Source: CAD feature listing. Evaluate the final solid. Frame: model axes, mm. A direction names the side the tool comes from. Round coordinates to 2 decimals unless told otherwise and drop trailing zeros. Write each loop counter-clockwise with the first axis right and the second up, starting at its lowest first coordinate (ties: lowest second). Pieces come first, ordered by that corner, then holes. Notation, with made-up numbers: M 42,87.5 L 46,87.5 A20 ccw 46,93.5 Z; hole C 78,-13.75 d3. An arc over 180 degrees is marked long. Use a Markdown table: item, result.
Autodesk Inventor part; units mm, degrees
ref_plane "YZ Plane" through (0, 0, 0) normal (1, 0, 0) x (0, 1, 0)
ref_plane "XZ Plane" through (0, 0, 0) normal (0, 1, 0) x (-1, 0, 0)
ref_plane "XY Plane" through (0, 0, 0) normal (0, 0, 1) x (1, 0, 0)
sketch "Sketch1" plane through (0, 0, 0) normal (0, 1, 0) x (-1, 0, 0)
  line L0 (-15.7, 12.7) -> (15.7, 12.7)
  line L1 (15.7, 12.7) -> (15.7, -12.7)
  line L2 (15.7, -12.7) -> (-15.7, -12.7)
  line L3 (-15.7, -12.7) -> (-15.7, 12.7)
  line L4 (-15.7, 12.7) -> (15.7, -12.7) construction
  line L5 (15.7, 12.7) -> (-15.7, -12.7) construction
  point P0 (0, 0)
  dimension "d0" = 25.4
  dimension "d1" = 31.4
extrude "Extrusion1" add sketch "Sketch1" along normal mid plane 6
sketch "Sketch2" plane through (0, 3, 0) normal (0, 1, 0) x (1, 0, 0)
  point P0 (0, 0)
hole "Hole1" at (0, 3, 0) direction (0, -1, 0) diameter 4.496 end through all
sketch "Sketch3" plane through (0, 3, 0) normal (0, 1, 0) x (1, 0, 0)
  circle A0 centre (0, 0) radius 3.875
  dimension "d11" = 7.75
extrude "Extrusion2" cut sketch "Sketch3" against normal blind 4.2672
sketch "Sketch4" plane through (0, 3, 0) normal (0, 1, 0) x (1, 0, 0)
  circle A0 centre (5.2, -7.7) radius 3.048
  line L0 (-15.7, -12.7) -> (15.7, -12.7) construction
  line L1 (15.7, -12.7) -> (15.7, 12.7) construction
  point P0 (0, 0)
  dimension "d14" = 6.096
  dimension "d18" = 5
  dimension "d23" = 10.5
extrude "Extrusion3" add sketch "Sketch4" along normal blind 4.572
sketch "Sketch5" plane through (0, -3, 0) normal (0, -1, 0) x (1, 0, 0)
  line L0 (-15.7, 12.7) -> (15.7, 12.7)
  line L1 (15.7, 12.7) -> (12.7, 12.7)
  line L2 (12.7, 12.7) -> (12.7, -12.7)
  line L3 (12.7, -12.7) -> (15.7, -12.7)
  line L4 (15.7, -12.7) -> (15.7, 12.7)
  line L5 (-15.7, 12.7) -> (-12.7, 12.7)
  line L6 (-12.7, 12.7) -> (-12.7, -12.7)
  line L7 (-12.7, -12.7) -> (-15.7, -12.7)
  line L8 (-15.7, -12.7) -> (-15.7, 12.7)
  line L9 (-15.7, -12.7) -> (15.7, -12.7)
  line L10 (12.7, 0) -> (-12.7, 0) construction
  point P0 (0, 0)
  point P1 (0, 0)
  dimension "d20" = 25.4
extrude "Extrusion4" add sketch "Sketch5" along normal blind 5 contours L0 L6 L7 L8 | L0 L4 L3 L2
fillet "Fillet1" radius 2 4 edges at (-15.7, -2.5, 12.7) (15.7, -2.5, 12.7) (15.7, -2.5, -12.7) (-15.7, -2.5, -12.7)
properties part number "BearingMount"
Q1. Section B-B on x = 5.2. Return loops of the section in (y, z), plus the area to 3 significant figures.
Results are:
| item | result |
|---|---|
| outline | M -3,-12.7 L 3,-12.7 L 3,4.65 L 7.57,4.65 L 7.57,10.75 L 3,10.75 L 3,12.7 L -3,12.7 Z |
| area | 180 mm^2 |
Q2. Section C-C on y = -0.25. Return loops of the section in (x, z) (3 decimals), plus the area to 3 significant figures.
Results are:
| item | result |
|---|---|
| outline | M -15.7,-10.7 A2 ccw -13.7,-12.7 L 13.7,-12.7 A2 ccw 15.7,-10.7 L 15.7,10.7 A2 ccw 13.7,12.7 L -13.7,12.7 A2 ccw -15.7,10.7 Z; hole C 0,0 d7.75 |
| area | 747 mm^2 |
Q3. Section A-A on z = 0. Return loops of the section in (x, y) (3 decimals), plus the area to 3 significant figures.
Results are:
| item | result |
|---|---|
| outline | M -15.7,-8 L -12.7,-8 L -12.7,-3 L -2.248,-3 L -2.248,-1.267 L -3.875,-1.267 L -3.875,3 L -15.7,3 Z; M 2.248,-3 L 12.7,-3 L 12.7,-8 L 15.7,-8 L 15.7,3 L 3.875,3 L 3.875,-1.267 L 2.248,-1.267 Z |
| area | 178 mm^2 |
Q4. First-contact query: pin 1 Ø12 at (x, z) = (-7, -5.5) entering from -Y; pin 2 Ø8.5 at (x, z) = (1.5, 0) entering from +Y; pin 3 Ø7 at (x, z) = (0, 0) entering from +Y; pin 4 Ø12.5 at (x, z) = (-1.5, 5.5) entering from -Y. Flat tips, straight axial feed; report the tip coordinate or a pass-through.
Results are:
| item | result |
|---|---|
| pin 1 | y = -8 |
| pin 2 | y = 3 |
| pin 3 | y = -1.27 |
| pin 4 | y = -3 |
Q5. Reachability of faces 5 (the flat face through (-12.7, -5, 0)), 6 (the cylindrical face through (2.953, 5.254, 9.76)), 7 (the cylindrical face through (15.13, -2.42, -12.1)) from +Z, -Z, +X, -X, +Y, -Y: full face, straight path, thin tool, end or side. Return the list, or none.
Results are:
| item | result |
|---|---|
| face 5 | +Z, -Z, -Y |
| face 6 | +Y |
| face 7 | -Z, +X, +Y, -Y |
Q6. Section D-D on x = -0.5. Return loops of the section in (y, z), plus the area to 3 significant figures.
Results are:
| item | result |
|---|---|
| outline | M -3,-12.7 L 3,-12.7 L 3,-3.84 L -1.27,-3.84 L -1.27,-2.19 L -3,-2.19 Z; M -3,2.19 L -1.27,2.19 L -1.27,3.84 L 3,3.84 L 3,12.7 L -3,12.7 Z |
| area | 112 mm^2 |
Q7. Line query: L1, parallel to X at y = -2, z = 0; L2, parallel to Z at x = 0, y = -1.85; L3, parallel to Z at x = 0, y = 0.3 (3 decimals). Output: solid intervals per line, ascending.
Results are:
| item | result |
|---|---|
| L1 | -15.7 to -2.25, 2.25 to 15.7 |
| L2 | -12.7 to -2.25, 2.25 to 12.7 |
| L3 | -12.7 to -3.875, 3.875 to 12.7 |
Q8. Mould query, pull axis Z, two halves, no side actions, for faces 1 (the flat face through (0, 0, -12.7)), 2 (the flat face through (0, 0, 12.7)), 3 (the cylindrical face through (1.37, -2.15, -1.78)), 4 (the flat face through (2, -1.267, 2)). Classes: +Z half, -Z half, draft (parallel to the pull), parting line (faces both ways), or undercut.
Results are:
| item | result |
|---|---|
| face 1 | -Z half |
| face 2 | +Z half |
| face 3 | undercut |
| face 4 | undercut |
